```python
from build123d import *

# Parameters (mm, degrees)
CYLINDER003_R     = 1
CYLINDER003_DEPTH = 10
ARRAY_COUNT       = 8
CYLINDER002_R     = 1.8
CYLINDER002_DEPTH = 1.5
CYLINDER001_R     = 1.7
CYLINDER001_DEPTH = 1.5
CYLINDER004_R     = 1
CYLINDER004_DEPTH = 10
CYLINDER_R        = 19
CYLINDER_DEPTH    = 10


with BuildPart() as array:
    # Cylinder003 → Cylinder003 (new body)
    with BuildSketch(Plane(origin=(-15, 0, 0), x_dir=(1, 0, 0), z_dir=(0, 0, 1))):
        Circle(CYLINDER003_R)
    extrude(amount=CYLINDER003_DEPTH)

    # Array: Array ×8 about axis
    array_axis = Axis((0, 0, 0), (0, 0, 1))


with BuildPart() as array_1:
    add(array.part)
    for i in range(1, ARRAY_COUNT):
        add(array.part.rotate(array_axis, i * 360 / ARRAY_COUNT))


with BuildPart() as recess1:
    # Cylinder002 → Cylinder002 (new body)
    with BuildSketch(Plane(origin=(-5, 0, 8.5), x_dir=(1, 0, 0), z_dir=(0, 0, 1))):
        Circle(CYLINDER002_R)
    extrude(amount=CYLINDER002_DEPTH)


with BuildPart() as recess2:
    # Cylinder001 → Cylinder001 (new body)
    with BuildSketch(Plane(origin=(5, 0, 8.5), x_dir=(1, 0, 0), z_dir=(0, 0, 1))):
        Circle(CYLINDER001_R)
    extrude(amount=CYLINDER001_DEPTH)


with BuildPart() as fusion:
    # Cylinder004 → Cylinder004 (new body)
    with BuildSketch(Plane(origin=(0, -4, 0), x_dir=(1, 0, 0), z_dir=(0, 0, 1))):
        Circle(CYLINDER004_R)
    extrude(amount=CYLINDER004_DEPTH)

    # Fusion: union Array, Recess1, Recess2
    add(array_1.part)
    add(recess1.part)
    add(recess2.part)


with BuildPart() as cut:
    # Cylinder → Cylinder (new body)
    with BuildSketch(Plane.XY):
        Circle(CYLINDER_R)
    extrude(amount=CYLINDER_DEPTH)

    # Cut: cut Fusion
    add(fusion.part, mode=Mode.SUBTRACT)


solid = cut.part
```
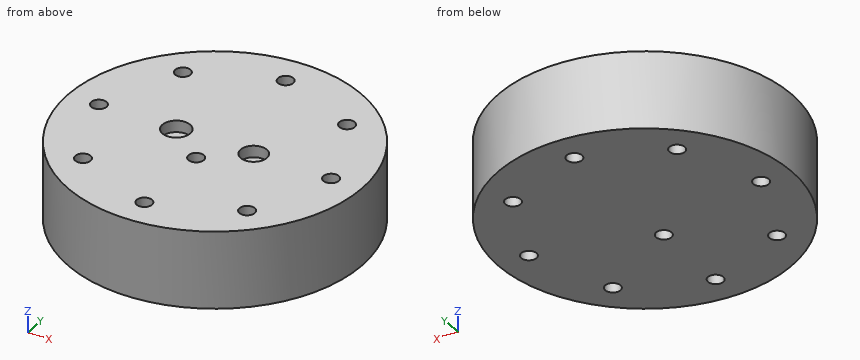
Check sheet for the modelled part. Datum: model origin and axes. Units: mm. Round coordinates to 2 decimals unless told otherwise and drop trailing zeros. Loops run counter-clockwise (first coordinate to the right, second up) from the corner with the lowest first, then second, coordinate; pieces in that order, holes last. Notation, with made-up numbers: (33.5, 69) -> (86.5, 69) arc R15 ccw to (86.5, 96) -> close; hole circle Ø7 at (3, -17). An arc over 180 degrees is marked (long way). Write item = value, one per line. Start each with the question number.
1) Sectioned sample at C-C, the plane y = -4. Record the cut outline in (x, z).
2) Sectioned sample at A-A, the plane y = 0. Record the cut outline in (x, z).
3) Sectioned sample at D-D, the plane z = 3.75. State how many separate pieces and enclosed holes the cut face has, plus the area to 3 significant figures.
4) Gauge pin test, flat ends, axial feed: pin 1 Ø1.6 at (x, y) = (15, 0) entering from +Z; pin 2 Ø3 at (x, y) = (-15, 0) entering from -Z; pin 3 Ø1.7 at (x, y) = (5, -0.5) entering from +Z; pin 4 Ø6 at (x, z) = (15, 2.5) entering from +Y. Record the tip position at first contact, or that the pin passes through.
5) Thickness scan on probe 1 along X at (y, z) = (-15, 3); probe 2 along Y at (x, z) = (-15.5, 5); probe 3 along Y at (x, z) = (7, 7.25). Record the ranges inside material, lowest first.
6) Sectioned sample at B-B, the plane x = 0. Record the cut outline in (y, z).
Results are:
q1.outline = (-18.57, 0) -> (-1, 0) -> (-1, 10) -> (-18.57, 10) -> close; (1, 0) -> (18.57, 0) -> (18.57, 10) -> (1, 10) -> close
q2.outline = (-19, 0) -> (-16, 0) -> (-16, 10) -> (-19, 10) -> close; (-14, 0) -> (14, 0) -> (14, 10) -> (6.7, 10) -> (6.7, 8.5) -> (3.3, 8.5) -> (3.3, 10) -> (-3.2, 10) -> (-3.2, 8.5) -> (-6.8, 8.5) -> (-6.8, 10) -> (-14, 10) -> close; (16, 0) -> (19, 0) -> (19, 10) -> (16, 10) -> close
q3.separate_pieces = 1
q3.enclosed_holes = 9
q3.area = 1,110 mm^2
q4.pin_1 = through
q4.pin_2 = 0
q4.pin_3 = 8.5
q4.pin_4 = 14.73
q5.probe_1 = -11.66 to -1, 1 to 11.66
q5.probe_2 = -10.99 to -0.87, 0.87 to 10.99
q5.probe_3 = -17.66 to 17.66
q6.outline = (-19, 0) -> (-16, 0) -> (-16, 10) -> (-19, 10) -> close; (-14, 0) -> (-5, 0) -> (-5, 10) -> (-14, 10) -> close; (-3, 0) -> (14, 0) -> (14, 10) -> (-3, 10) -> close; (16, 0) -> (19, 0) -> (19, 10) -> (16, 10) -> close
